Drawing for the job (mm, zero at the part's lowest x, y, z). Give positions to 0.01 mm unless a question says otherwise; leave off trailing zeros. Write each loop counter-clockwise with the first axis right and the second up, starting at its lowest first coordinate (ties: lowest second). Pieces come first, ordered by that corner, then holes. Notation, with made-up numbers: M 76.25,71.5 L 126.25,71.5 A21 ccw 126.25,84.5 Z; hole C -20,40.5 d6. An arc over 180 degrees is marked long. Answer as a JSON object with one key per item and string values. Group by question number.
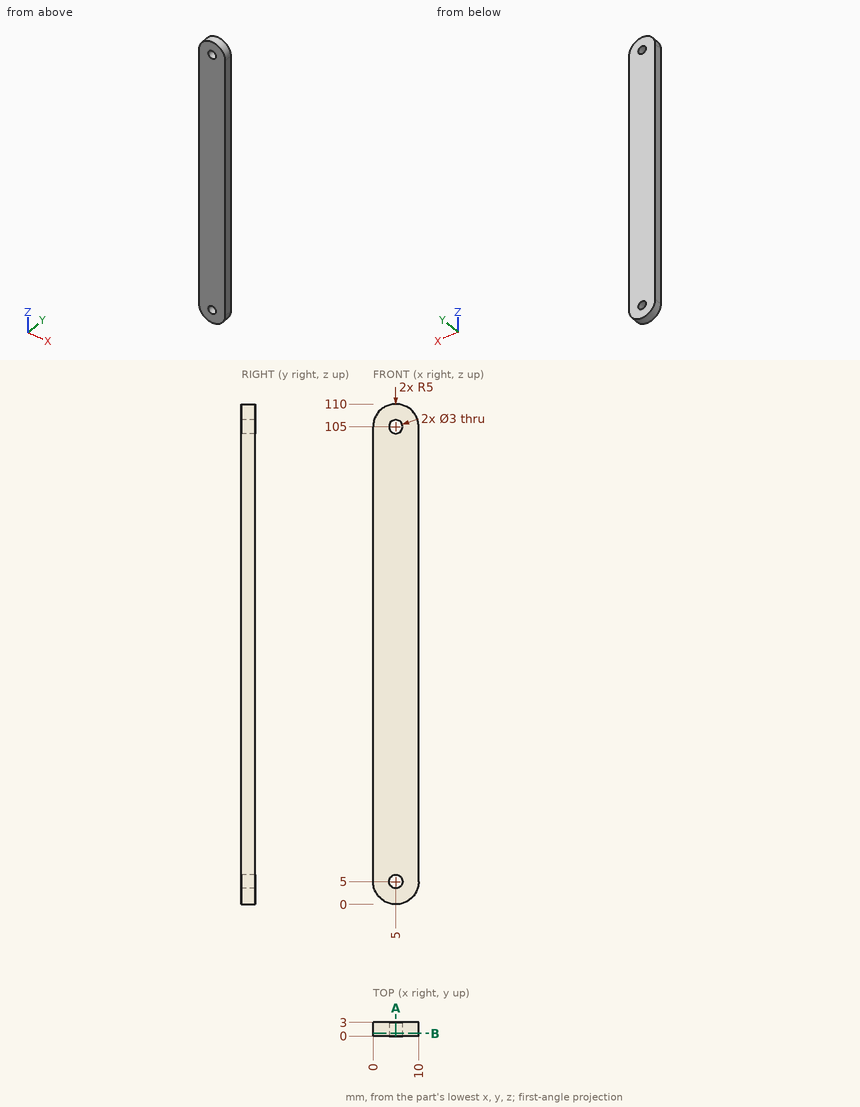
Q1. Slice it at A-A, the plane x = 5. Write the cut outline in (y, z).
Q2. Wall check: L1, parallel to Z at x = 5, y = 1.05; L2, parallel to X at y = 1.1, z = 105; L3, parallel to Z at x = 4.5, y = 2.5. Give the ranges that are in metal, low to high.
Q3. Slice it at B-B, the plane y = 0.6. Write the cut outline in (x, z), then the cut area to 3 significant figures.
Q4. Drop a flat-ended pin along its axis: P1, Ø1.5, axis at x = 8, y = 0.5, coming from the -Z side. Give the stop position or say it passes through.
Solved:
{
 "1": {"outline": "M 0,0 L 3,0 L 3,3.5 L 0,3.5 Z; M 0,6.5 L 3,6.5 L 3,103.5 L 0,103.5 Z; M 0,106.5 L 3,106.5 L 3,110 L 0,110 Z"},
 "2": {"L1": "z = 0 to 3.5, 6.5 to 103.5, 106.5 to 110", "L2": "x = 0 to 3.5, 6.5 to 10", "L3": "z = 0.03 to 3.59, 6.41 to 103.59, 106.41 to 109.97"},
 "3": {"outline": "M 0,5 A5 ccw 10,5 L 10,105 A5 ccw 0,105 Z; hole C 5,5 d3; hole C 5,105 d3", "area": "1,060 mm²"},
 "4": {"P1": "stops at z = 0.53"}
}
